Source: CAD feature listing. Evaluate the final solid. Frame: model axes, mm. A direction names the side the tool comes from. Round coordinates to 2 decimals unless told otherwise and drop trailing zeros. Order: outer loops, then holes, each group sorted by start corner. A loop starts at its lowest first (then second) coordinate and runs counter-clockwise, first axis right, second up. Notation, with made-up numbers: (76, -3) -> (129, -3) arc R9 cw to (129, 13) -> close; hole circle Ø8 at (61.25, 16). An arc over 180 degrees is marked (long way). One line per item, written item: value. Start each with the question number.
1) Reachability of faces 1 (the face through (-0.13, 3.99, 0.75)), 2 (the face through (-0.1, 1.2, 0)) from +Z, -Z, +X, -X, +Y, -Y: full face, straight path, thin tool, end or side. Return the list, or none.
2) Pin query (flat end, axial travel): P1, Ø1.6, axis at x = -2.6, y = -1.5, coming from the +Z side. Return the tip coordinate at first contact, or that it passes through.
3) Mould query, pull axis Y, two halves, no side actions, for faces 3 (the face through (3, 2, 0.5)), 4 (the face through (-1.2, 0.1, 1)), 5 (the face through (-1.08, -4.88, 0.49)), 6 (the face through (-0.217, -0.976, 0.507)). Classes: pulls with the +Y half, pulls with the -Y half, needs draft (parallel to the pull), parting line crosses it, or undercut.
4) Section A-A (y = 0). Return the cut outline in (x, z).
5) Section B-B (x = 0). Return the cut outline in (y, z), and give its area (3 significant figures).
6) Ray query, L1, parallel to Y at x = 0, z = 0.9; L2, parallel to Y at x = 0, z = 0.4; L3, parallel to Y at x = 1.75, z = 0.95. Return the intervals inside material, ascending.
7) Section D-D (y = 3). Return the cut outline in (x, z), and give its area (3 significant figures).
8) Section C-C (z = 0.7). Return the cut outline in (x, y).
```python
from build123d import *

# Parameters (mm, degrees)
F0_R     = 5
F1_DEPTH = 1
F2_R     = 1
F3_DEPTH = 0.5
F4_R     = 1
F5_DEPTH = 1


with BuildPart() as f1:
    # F0 (on Top) → F1 (new body)
    with BuildSketch(Plane.XY):
        Circle(F0_R)
    extrude(amount=F1_DEPTH)

    # F2 (on face) → F3 (cut)
    with BuildSketch(Plane.XY.offset(1)):
        with Locations((0, 3)):
            Circle(F2_R)
        with Locations((-2.598076, 1.5)):
            Circle(F2_R)
        with Locations((-2.598076, -1.5)):
            Circle(F2_R)
        with Locations((0, -3)):
            Circle(F2_R)
        with Locations((2.598076, -1.5)):
            Circle(F2_R)
        with Locations((2.598076, 1.5)):
            Circle(F2_R)
    extrude(amount=-F3_DEPTH, mode=Mode.SUBTRACT)

    # F4 (on face) → F5 (cut)
    with BuildSketch(Plane.XY.offset(1)):
        Circle(F4_R)
    extrude(amount=-F5_DEPTH, mode=Mode.SUBTRACT)


solid = f1.part
```
Findings:
1. face 1: +Z
1. face 2: -Z, +X, -X, +Y, -Y
2. P1: z = 0.5
3. face 3: undercut
3. face 4: needs draft
3. face 5: parting line crosses it
3. face 6: undercut
4. outline: (-5, 0) -> (-1, 0) -> (-1, 1) -> (-5, 1) -> close; (1, 0) -> (5, 0) -> (5, 1) -> (1, 1) -> close
5. outline: (-5, 0) -> (-1, 0) -> (-1, 1) -> (-2, 1) -> (-2, 0.5) -> (-4, 0.5) -> (-4, 1) -> (-5, 1) -> close; (1, 0) -> (5, 0) -> (5, 1) -> (4, 1) -> (4, 0.5) -> (2, 0.5) -> (2, 1) -> (1, 1) -> close
5. area: 6.00 mm2
6. L1: -5 to -4, -2 to -1, 1 to 2, 4 to 5
6. L2: -5 to -1, 1 to 5
6. L3: -4.68 to -2.03, -0.97 to 0.97, 2.03 to 4.68
7. outline: (-4, 0) -> (4, 0) -> (4, 1) -> (1, 1) -> (1, 0.5) -> (-1, 0.5) -> (-1, 1) -> (-4, 1) -> close
7. area: 7.00 mm2
8. outline: circle Ø10 at (0, 0); hole circle Ø2 at (-2.6, -1.5); hole circle Ø2 at (-2.6, 1.5); hole circle Ø2 at (0, -3); hole circle Ø2 at (0, 0); hole circle Ø2 at (0, 3); hole circle Ø2 at (2.6, -1.5); hole circle Ø2 at (2.6, 1.5)
